For this review, take the finished solid that the model builds, in its own axes (mm). Give positions to 0.01 mm unless a question says otherwise; leave off trailing zeros. Write each loop counter-clockwise with the first axis right and the second up, starting at its lowest first coordinate (ties: lowest second). Pieces come first, ordered by that corner, then holes. Notation, with made-up numbers: (-1, 43.25) -> (42, 43.25) arc R20 ccw to (42, 66.25) -> close; hole circle Ø5 at (-28.5, -14). An arc over 180 degrees is marked (long way). Write item = value, one per line.
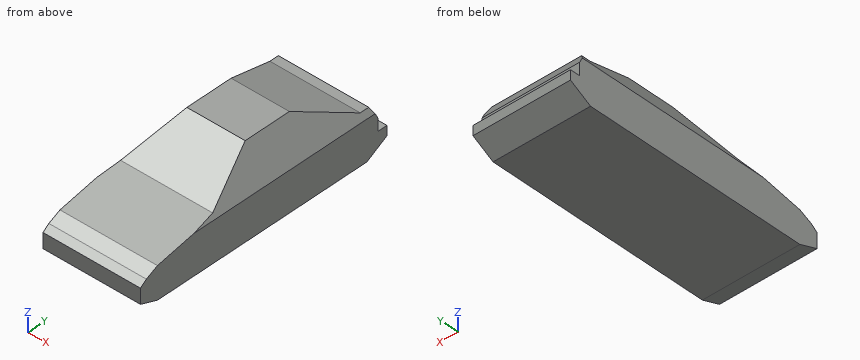
```python
from build123d import *

# Parameters (mm, degrees)
F1_DEPTH = 150.622
F3_START = 88.392
F3_DEPTH = 114.1679836892


with BuildPart() as f1:
    # F0 (on Front) → F1 (new body)
    with BuildSketch(Plane.XZ):
        Polygon((-25.7749836892, 0), (0, 0), (25.7749836892, 0), (25.7749836892, 24.2791596506), (6.3844995154, 56.1167374253), (0, 56.1167374253), (-6.3844995154, 56.1167374253), (-25.7749836892, 24.2791596506), align=None)
    extrude(amount=F1_DEPTH)

    # F2 (on Right) → F3 (intersect)
    with BuildSketch(Plane.YZ.offset(F3_START)):
        Polygon((-151.6052931547, 13.9350751415), (-151.6052931547, 7.0942197926), (-140.8825235742, 3.293744754), (-21.8824129552, 3.293744754), (-10.4809878394, 9.627870284), (-10.4809878394, 14.6951703355), (-15.693005628, 14.6951703355), (-15.693005628, 21.3516374031), (-18.8420340419, 27.3634195328), (-23.6559715122, 27.3634195328), (-54.8198632896, 41.2984937429), (-79.972098349, 41.2984937429), (-108.0265119672, 26.6033262014), (-140.9639567137, 20.2692002058), (-147.2980827093, 17.2288194299), align=None)
    extrude(amount=-F3_DEPTH, mode=Mode.INTERSECT)


solid = f1.part
```
(1) Take a section at D-D (y = -42). Write out the cut boundary in (x, z).
Answers below:
outline = (-25.77, 3.29) -> (25.77, 3.29) -> (25.77, 24.28) -> (18.9, 35.57) -> (-18.9, 35.57) -> (-25.77, 24.28) -> close
(2) Take a section at C-C (x = -4). Write out the cut boundary in (y, z), plus the area to 3 significant figures.
Answers below:
outline = (-150.62, 6.75) -> (-140.88, 3.29) -> (-21.88, 3.29) -> (-10.48, 9.63) -> (-10.48, 14.7) -> (-15.69, 14.7) -> (-15.69, 21.35) -> (-18.84, 27.36) -> (-23.66, 27.36) -> (-54.82, 41.3) -> (-79.97, 41.3) -> (-108.03, 26.6) -> (-140.96, 20.27) -> (-147.3, 17.23) -> (-150.62, 14.69) -> close
area = 3,780 mm^2
(3) Take a section at B-B (y = -76.5). Write out the cut boundary in (x, z), plus the area to 3 significant figures.
Answers below:
outline = (-25.77, 3.29) -> (25.77, 3.29) -> (25.77, 24.28) -> (15.41, 41.3) -> (-15.41, 41.3) -> (-25.77, 24.28) -> close
area = 1,780 mm^2
(4) For pin 1 (3 mm diameter, centred on x = 1.5, z = 20, fed in from -Y); pin 2 (1.5 mm diameter, centred on x = -16.5, z = 29.5, fed in from -Y); pin 3 (1.4 mm diameter, centred on x = -3.5, y = -21, fed in from +Z), all flat-tipped, find the tip position at first contact; note any pin that passes through.
Answers below:
pin_1 = -144.65
pin_2 = -103.93
pin_3 = 27.36
(5) Take a section at A-A (x = -20.5). Write out the cut boundary in (y, z), plus the area to 3 significant figures.
Answers below:
outline = (-150.62, 6.75) -> (-140.88, 3.29) -> (-21.88, 3.29) -> (-10.48, 9.63) -> (-10.48, 14.7) -> (-15.69, 14.7) -> (-15.69, 21.35) -> (-18.84, 27.36) -> (-23.66, 27.36) -> (-36.13, 32.94) -> (-95.93, 32.94) -> (-108.03, 26.6) -> (-140.96, 20.27) -> (-147.3, 17.23) -> (-150.62, 14.69) -> close
area = 3,420 mm^2
(6) To check wall thickness, follow probe 1 along Z at (x, y) = (22, -23); probe 2 along Z at (x, y) = (-4, -103); probe 3 along Y at (x, z) = (-1.5, 37.5). State the ranges of each line that lie inside material, in increasing order.
Answers below:
probe_1 = 3.29 to 27.36
probe_2 = 3.29 to 29.24
probe_3 = -87.22 to -46.33
